from build123d import *

# Parameters (mm, degrees)
F0_R     = 4
F1_DEPTH = 70
F3_DEPTH = 8
F4_W     = 4.341884
F4_H     = 1.508987
F5_DEPTH = 5


with BuildPart() as f1:
    # F0 (on Front) → F1 (new body)
    with BuildSketch(Plane.XZ):
        Circle(F0_R)
    extrude(amount=F1_DEPTH)

    # F2 (on face) → F3 (join)
    with BuildSketch(Plane.XZ.offset(70)):
        Polygon((4.341884, -7.4932), (8.660243, 0.013582), (4.31836, 7.506782), (-4.341884, 7.4932), (-8.660243, -0.013582), (-4.31836, -7.506782), align=None)
    extrude(amount=F3_DEPTH)

    # F4 (on face) → F5 (join)
    with BuildSketch(Plane.XZ.offset(78)):
        with Locations((2.170942, -0.754493)):
            Rectangle(F4_W, F4_H)
    extrude(amount=F5_DEPTH)

    # F6 (on face) → F7 (revolve)
    with BuildSketch(Plane.XY):
        Polygon((4.341884, -83), (0, -83), (0, -86), (10, -94), (25, -94), (8, -78), (4.341884, -78), align=None)
    revolve(axis=Axis((0, -86, 0), (0, -1, 0)))


solid = f1.part
Could you check a few things on this model? Use its own coordinates, in mm. A direction names the side the tool comes from. Coordinates: 2 decimals unless noted, no trailing zeros. Write each loop counter-clockwise with the first axis right and the second up, starting at its lowest first coordinate (ties: lowest second). Pieces come first, ordered by that corner, then holes. Notation, with made-up numbers: M 87,16.5 L 145,16.5 A30 cw 145,55.5 Z; hole C 0.5,47.5 d10. An arc over 180 degrees is marked long. One line per question, with ' | ' between items.
1) If we mould it in two halves opening along Z, with no side actions, what happens to faces 1 (the face through (-0.376, -87.389, -1.695)), 2 (the face through (2, -80, 0)), 3 (the face through (6.52, -73.94, 3.71)), 4 (the face through (6.7, -78, 3.8))? For each: released by +Z, released by -Z, zero draft, split by the parting line, or undercut.
Checks:
face 1: undercut | face 2: undercut | face 3: released by +Z | face 4: zero draft
2) For faces 5 (the face through (-6.47, -73.94, 3.79)), 6 (the face through (-6.7, -78, -3.9)), 7 (the face through (-0.867, -34.51, -3.905)), which set-ups out of +Z, -Z, +X, -X, +Y, -Y let a thin tool reach every point of the face, with its end or its side?
Checks:
face 5: +Z, -X, +Y | face 6: -Z, -X, +Y | face 7: +Y
3) I need wall thicknesses on probe 1 along X at (y, z) = (-63, 2.5); probe 2 along Y at (x, z) = (-0.5, 15); probe 3 along Y at (x, z) = (14, 4). Which ranges of each line are inside material? Lowest first, please. Write a range as [from, to].
Checks:
probe 1: [-3.12, 3.12] | probe 2: [-94, -84.6] | probe 3: [-94, -84.17]
4) For pin 1 Ø7 at (x, z) = (-0.5, -2) entering from -Y; pin 2 Ø12 at (x, y) = (5.5, -24) entering from +Z; pin 3 Ø1.5 at (x, z) = (-3.5, 7) entering from -Y, each with a flat end and sliding along its axis, tell me the tip position at first contact or that it passes through.
Checks:
pin 1: y = -90.45 | pin 2: z = 4 | pin 3: y = -92.86
5) Imagine slicing it at A-A, the plane y = -9. Write out the boundary of the cut face in (x, z).
Checks:
outline: C 0,0 d8
